Check sheet for the drawn part. Datum: minimum x, y, z corner. Units: mm. Round coordinates to 2 decimals unless told otherwise and drop trailing zeros. Write each loop counter-clockwise with the first axis right and the second up, starting at its lowest first coordinate (ties: lowest second). Pieces come first, ordered by that corner, then holes. Notation, with made-up numbers: (44.5, 33.5) - (90.5, 33.5) arc R16 cw to (90.5, 41.5) - close; hole circle Ø9 at (7, 70). An arc over 180 degrees is marked (long way). Answer as a JSON object with one key per item and string values. Group by question number.
1) Section check B-B (x = 14). Enter the section's corners in (y, z), then the cut area to 3 significant figures.
2) Go/stop test with flat-tipped pins: pin 1 Ø2 at (y, z) = (24.5, 2) entering from -X; pin 2 Ø2 at (x, z) = (14.5, 2.5) entering from -Y; pin 3 Ø1.2 at (y, z) = (21, 2) entering from +X. Record where each tip stops, or that it passes through.
3) Thickness scan on line 1 (Y direction, x = 27, z = 3.4); line 2 (Y direction, x = 23.76, z = 3); line 3 (Y direction, x = 17.5, z = 3.2). Record the ranges inside material, lowest first.
4) Section check A-A (x = 6.76). Enter the section's corners in (y, z).
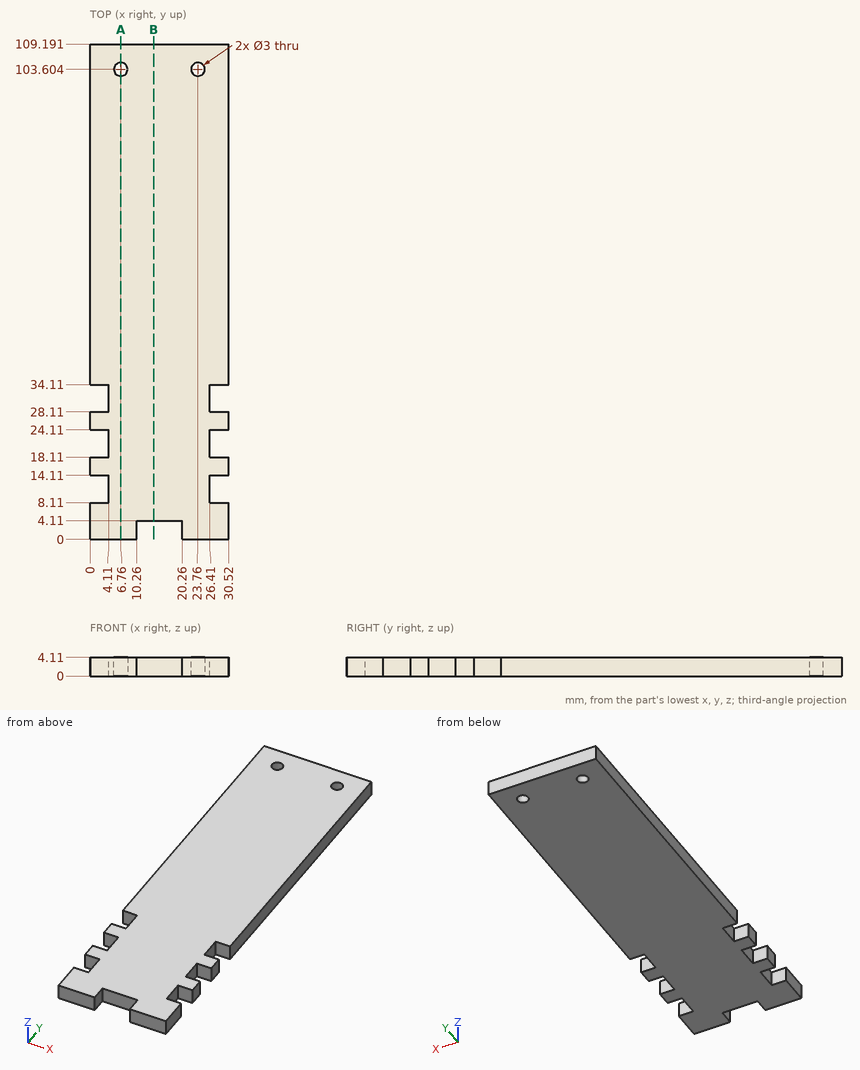
Returned:
{
 "1": {"outline": "(4.11, 0) - (109.19, 0) - (109.19, 4.11) - (4.11, 4.11) - close", "area": "432 mm2"},
 "2": {"pin 1": "x = 0", "pin 2": "y = 4.11", "pin 3": "x = 26.41"},
 "3": {"line 1": "0 to 8.11, 14.11 to 18.11, 24.11 to 28.11, 34.11 to 109.19", "line 2": "0 to 102.1, 105.1 to 109.19", "line 3": "4.11 to 109.19"},
 "4": {"outline": "(0, 0) - (102.1, 0) - (102.1, 4.11) - (0, 4.11) - close; (105.1, 0) - (109.19, 0) - (109.19, 4.11) - (105.1, 4.11) - close"}
}
